```python
from build123d import *

# Parameters (mm, degrees)
SKETCH1_W            = 127
SKETCH1_H            = 152.4
BOSS_EXTRUDE1_DEPTH  = 10
SKETCH2_W            = 25.4
SKETCH2_H            = 7.9375
CUT_EXTRUDE1_DEPTH   = 10
LPATTERN1_COUNT      = 2
LPATTERN1_PITCH      = 76.2
LPATTERN1_COUNT_DIR2 = 2
LPATTERN1_PITCH_DIR2 = 88.9
SKETCH3_R            = 3.175
CUT_EXTRUDE2_DEPTH   = 10
LPATTERN2_COUNT      = 2
LPATTERN2_PITCH      = 101.6
CUT_EXTRUDE3_DEPTH   = 10
LPATTERN3_COUNT      = 2
LPATTERN3_PITCH      = 101.6
FILLET1_R            = 12.7
FILLET2_R            = 12.7


with BuildPart() as part:
    # Sketch1 → Boss-Extrude1 (new body)
    with BuildSketch(Plane.XY):
        with Locations((-63.5, 76.2)):
            Rectangle(SKETCH1_W, SKETCH1_H)
    extrude(amount=BOSS_EXTRUDE1_DEPTH)

    # Sketch2 → Cut-Extrude1 (cut)
    with BuildSketch(Plane.XY.offset(10)):
        with Locations((-101.6, 122.22353)):
            Rectangle(SKETCH2_W, SKETCH2_H)
    cut_extrude1 = extrude(amount=-CUT_EXTRUDE1_DEPTH, mode=Mode.SUBTRACT)

    # LPattern1: Cut-Extrude1 2 × 2
    with Locations(*[(i * LPATTERN1_PITCH, -j * LPATTERN1_PITCH_DIR2, 0) for i in range(LPATTERN1_COUNT) for j in range(LPATTERN1_COUNT_DIR2) if (i, j) != (0, 0)]):
        add(cut_extrude1, mode=Mode.SUBTRACT)

    # Sketch3 → Cut-Extrude2 (cut)
    with BuildSketch(Plane.XY.offset(10)):
        with Locations((-114.3, 139.7)):
            Circle(SKETCH3_R)
    cut_extrude2 = extrude(amount=-CUT_EXTRUDE2_DEPTH, mode=Mode.SUBTRACT)

    # LPattern2: Cut-Extrude2 ×2
    with Locations(*[(i * LPATTERN2_PITCH, 0, 0) for i in range(1, LPATTERN2_COUNT)]):
        add(cut_extrude2, mode=Mode.SUBTRACT)

    # Sketch4 → Cut-Extrude3 (cut)
    with BuildSketch(Plane.XY.offset(10)):
        with BuildLine():
            Line((-110.32998, 17.6403), (-110.32998, 9.7028))
            ThreePointArc((-110.32998, 9.7028), (-114.3, 5.73278), (-118.27002, 9.7028))
            Line((-118.27002, 9.7028), (-118.27002, 17.6403))
            ThreePointArc((-118.27002, 17.6403), (-114.3, 21.61032), (-110.32998, 17.6403))
        make_face()
    cut_extrude3 = extrude(amount=-CUT_EXTRUDE3_DEPTH, mode=Mode.SUBTRACT)

    # LPattern3: Cut-Extrude3 ×2
    with Locations(*[(i * LPATTERN3_PITCH, 0, 0) for i in range(1, LPATTERN3_COUNT)]):
        add(cut_extrude3, mode=Mode.SUBTRACT)

    # Fillet1
    fillet1_edges = [part.edges().sort_by_distance(p)[0] for p in [
        (0, 152.4, 5),
    ]]
    fillet(fillet1_edges, radius=FILLET1_R)

    # Fillet2
    fillet2_edges = [part.edges().sort_by_distance(p)[0] for p in [
        (-127, 152.4, 5),
        (0, 0, 5),
        (-127, 0, 5),
    ]]
    fillet(fillet2_edges, radius=FILLET2_R)


solid = part.part
```
Here's how the part is built. I have some questions about the finished solid (model axes, mm). A direction names the side the tool comes from. Give positions to 0.01 mm unless a question says otherwise; leave off trailing zeros. Order: outer loops, then holes, each group sorted by start corner. A loop starts at its lowest first (then second) coordinate and runs counter-clockwise, first axis right, second up. Notation, with made-up numbers: (-35, -9.75) - (11, -9.75) arc R20 ccw to (11, 23.25) - close; hole circle Ø2 at (-6.5, 45). An arc over 180 degrees is marked (long way). Answer as a JSON object with one key per item and string values. Group by question number.
Item 1: If we section it at B-B on z = 8.5: Give the number of separate pieces and of enclosed holes in the cut face, and give its area (3 significant figures).
Item 2: If we section it at A-A on x = -103: Please give me the cut outline in (y, z).
Item 3: If we mould it in two halves opening along Y, with no side actions, what happens to faces 1 (the flat face through (-114.3, 122, 5)), 2 (the cylindrical face through (-3.62, 3.82, 5.07)), 3 (the flat face through (-64, 77, 10))? For each: pulls with the +Y half, pulls with the -Y half, needs draft (parallel to the pull), parting line crosses it, or undercut.
Item 4: Which directions (+Z, -Z, +X, -X, +Y, -Y) give clear straight access to the entire face, cutting with the end or side of a thin tool? Please do faces 4 (the flat face through (-64, 152.4, 5)), 5 (the flat face through (-102, 126.192, 5)).
Item 5: Please list where these lines run through material, in increasing order: probe 1 along Y at (x, z) = (-34, 7.25); probe 2 along X at (y, z) = (16.5, 3.25); probe 3 along Y at (x, z) = (-13, 1.5).
Result set:
{
 "1": {"separate pieces": "1", "enclosed holes": "8", "area": "18,100 mm²"},
 "2": {"outline": "(0, 0) - (29.35, 0) - (29.35, 10) - (0, 10) - close; (37.29, 0) - (118.25, 0) - (118.25, 10) - (37.29, 10) - close; (126.19, 0) - (152.4, 0) - (152.4, 10) - (126.19, 10) - close"},
 "3": {"face 1": "undercut", "face 2": "pulls with the -Y half", "face 3": "needs draft"},
 "4": {"face 4": "+Z, -Z, +X, -X, +Y", "face 5": "+Z, -Z"},
 "5": {"probe 1": "0 to 29.35, 37.29 to 118.25, 126.19 to 152.4", "probe 2": "-127 to -118.27, -110.33 to -16.67, -8.73 to 0", "probe 3": "0 to 5.74, 21.6 to 29.35, 37.29 to 118.25, 126.19 to 136.54, 142.86 to 152.4"}
}
